Check sheet for the modelled part. Datum: model origin and axes. Units: mm. A direction names the side the tool comes from. Round coordinates to 2 decimals unless told otherwise and drop trailing zeros. Order: outer loops, then holes, each group sorted by start corner. A loop starts at its lowest first (then second) coordinate and runs counter-clockwise, first axis right, second up.
from build123d import *

# Parameters (mm, degrees)
BOSS_EXTRUDE1_DEPTH = 97.3582
SKETCH5_W           = 11.10345239
SKETCH5_H           = 12.145052052
SKETCH5_R           = 3.8481
CUT_EXTRUDE2_DEPTH  = 0.4445
SKETCH6_W           = 10.752068687
SKETCH6_H           = 11.509710708
SKETCH6_R           = 3.8481
CUT_EXTRUDE3_DEPTH  = 0.4445
SKETCH7_W           = 11.973800556
SKETCH7_H           = 12.349285591
SKETCH7_R           = 3.8481
CUT_EXTRUDE4_DEPTH  = 0.4445
SKETCH8_W           = 12.812601238
SKETCH8_H           = 11.483340014
SKETCH8_R           = 3.8481
CUT_EXTRUDE5_DEPTH  = 0.4445
SKETCH9_W           = 15.274592148
SKETCH9_H           = 13.977564657
CUT_EXTRUDE6_DEPTH  = 3.683
SKETCH11_W          = 19.244818326
SKETCH11_H          = 17.400851683
CUT_EXTRUDE7_DEPTH  = 3.937


with BuildPart() as part:
    # Sketch1 → Boss-Extrude1 (new body)
    with BuildSketch(Plane.XY):
        Polygon((0, 5.499261314), (-4.7625, 2.749630657), (-4.7625, -2.749630657), (0, -5.499261314), (4.7625, -2.749630657), (4.7625, 2.749630657), align=None)
    extrude(amount=BOSS_EXTRUDE1_DEPTH)

    # Sketch5 → Cut-Extrude2 (cut, symmetric)
    with BuildSketch(Plane.XY.offset(79.0448)):
        with Locations((-0.378227241, -0.09440181)):
            Rectangle(SKETCH5_W, SKETCH5_H)
        Circle(SKETCH5_R, mode=Mode.SUBTRACT)
    extrude(amount=CUT_EXTRUDE2_DEPTH, both=True, mode=Mode.SUBTRACT)

    # Sketch6 → Cut-Extrude3 (cut, symmetric)
    with BuildSketch(Plane.XY.offset(65.5066)):
        with Locations((-0.265980709, -0.185380495)):
            Rectangle(SKETCH6_W, SKETCH6_H)
        Circle(SKETCH6_R, mode=Mode.SUBTRACT)
    extrude(amount=CUT_EXTRUDE3_DEPTH, both=True, mode=Mode.SUBTRACT)

    # Sketch7 → Cut-Extrude4 (cut, symmetric)
    with BuildSketch(Plane.XY.offset(89.8017)):
        with Locations((-0.368386295, 0.291901412)):
            Rectangle(SKETCH7_W, SKETCH7_H)
        Circle(SKETCH7_R, mode=Mode.SUBTRACT)
    extrude(amount=CUT_EXTRUDE4_DEPTH, both=True, mode=Mode.SUBTRACT)

    # Sketch8 → Cut-Extrude5 (cut, symmetric)
    with BuildSketch(Plane(origin=(0, 0, 7.3025), x_dir=(-1, 0, 0), z_dir=(0, 0, -1))):
        with Locations((-0.353342966, -0.03551845)):
            Rectangle(SKETCH8_W, SKETCH8_H)
        Circle(SKETCH8_R, mode=Mode.SUBTRACT)
    extrude(amount=CUT_EXTRUDE5_DEPTH, both=True, mode=Mode.SUBTRACT)

    # Sketch9 → Cut-Extrude6 (cut)
    with BuildSketch(Plane(origin=(0, 0, 0), x_dir=(-1, 0, 0), z_dir=(0, 0, -1))):
        with Locations((0.659891111, -0.649631618)):
            Rectangle(SKETCH9_W, SKETCH9_H)
    extrude(amount=-CUT_EXTRUDE6_DEPTH, mode=Mode.SUBTRACT)

    # Sketch11 → Cut-Extrude7 (cut)
    with BuildSketch(Plane.XY.offset(97.3582)):
        with Locations((0.649471759, -1.230390771)):
            Rectangle(SKETCH11_W, SKETCH11_H)
    extrude(amount=-CUT_EXTRUDE7_DEPTH, mode=Mode.SUBTRACT)


solid = part.part
1) Sectioned sample at A-A on z = 12.5. Record the cut outline in (x, y).
2) Set-up check for faces 1 (the face through (-4.762, 0, 92)), 2 (the face through (-0.834, -3.757, 89.795)): record each of +Z, -Z, +X, -X, +Y, -Y from which the full face is reachable in a straight line by a thin tool's end or side.
3) Scan lines: line 1 (Y direction, x = 1.25, z = 25); line 2 (Y direction, x = -1.75, z = 58); line 3 (X direction, y = -3.75, z = 51). Record each from-to range of solid material in increasing order.
4) Draft check along Z on faces 3 (the face through (2.348, -4.144, 72.187)), 4 (the face through (0, 0, 93.421)), 5 (the face through (2, -4, 78.6)). Enter one of: pulls with the +Z half, pulls with the -Z half, needs draft (parallel to the pull), parting line crosses it, or undercut.
Values found:
1. outline: (-4.76, -2.75) - (0, -5.5) - (4.76, -2.75) - (4.76, 2.75) - (0, 5.5) - (-4.76, 2.75) - close
2. face 1: +Z, -Z, -X, +Y, -Y
2. face 2: none
3. line 1: y = -4.78 to 4.78
3. line 2: y = -4.49 to 4.49
3. line 3: x = -3.03 to 3.03
4. face 3: needs draft
4. face 4: pulls with the +Z half
4. face 5: undercut
